Input: part model. Units: mm. Frame: model coordinates. Face numbers are marked on the shaded views. A direction names the side the tool comes from. Give positions to 0.01 mm unless a question says otherwise; leave off trailing zeros. Loops run counter-clockwise (first coordinate to the right, second up) from the corner with the lowest first, then second, coordinate; pieces in that order, holes last. Notation, with made-up numbers: (4.5, -14.5) - (24.5, -14.5) arc R9 ccw to (24.5, 0.5) - close; hole circle Ø5 at (30, 81). An arc over 180 degrees is marked (long way). Answer as a JSON object with one key per item and string values. Group by question number.
(1) Section query A-A (z = -522.75). Return loops of the section in (x, y), plus the area to 3 significant figures.
(2) Access query for the marked faces 4 and 5. Directions: +Z, -Z, +X, -X, +Y, -Y. A direction counts if a zero-diameter tool reaches every point of the face in a straight line with its end or side. Return the directions, or none.
(3) Pin query (flat end, axial travel): P1, Ø1.5, axis at y = 596, z = -512.5, coming from the +X side; P2, Ø4.5, axis at x = -734.753, z = -516, coming from the -Y side. Return the tip coordinate at first contact, or that it passes through.
(4) Section query C-C (x = -759.5). Return loops of the section in (y, z), plus the area to 3 significant figures.
(5) Section query B-B (y = 595). Return loops of the section in (x, z), plus the area to 3 significant figures.
(6) Mould query, pull axis X, two halves, no side actions, for the marked faces 1, 2 and 3. Classes: +X half, -X half, draft (parallel to the pull), parting line (faces both ways), or undercut.
(7) Section query D-D (z = -516). Return loops of the section in (x, y).
(8) Material intervals for L1, parallel to X at y = 594.95, z = -521.75; L2, parallel to X at y = 596.7, z = -516; L3, parallel to X at y = 595.7, z = -517.5, sorted ascending.
```python
from build123d import *

# Parameters (mm, degrees)
BOX001_W        = 40
BOX001_H        = 4
BOX001_DEPTH    = 25
SKETCH002_R     = 2.5781
POCKET002_DEPTH = 4.001
FILLET_R        = 10


with BuildPart() as part:
    # Box001 → Box001 (new body)
    with BuildSketch(Plane(origin=(-768, 594, -530), x_dir=(1, 0, 0), z_dir=(0, 0, 1))):
        with Locations((20, 2)):
            Rectangle(BOX001_W, BOX001_H)
    extrude(amount=BOX001_DEPTH)

    # Sketch002 → Pocket002 (cut, through all)
    with BuildSketch(Plane(origin=(-768, 598, -530), x_dir=(-1, 0, 0), z_dir=(0, 1, 0))):
        with Locations((-33.247, 14)):
            Circle(SKETCH002_R)
        with Locations((-8.5, 14)):
            Circle(SKETCH002_R)
        with BuildLine():
            ThreePointArc((-13.7, 12), (-20.85, 19.15), (-28, 12))
            Line((-28, 12), (-28, 0))
            Line((-28, 0), (-13.7, 0))
            Line((-13.7, 12), (-13.7, 0))
        make_face()
    extrude(amount=-POCKET002_DEPTH, mode=Mode.SUBTRACT)

    # Fillet
    fillet_edges = [part.edges().sort_by_distance(p)[0] for p in [
        (-728, 596, -505),
    ]]
    fillet(fillet_edges, radius=FILLET_R)


solid = part.part
```
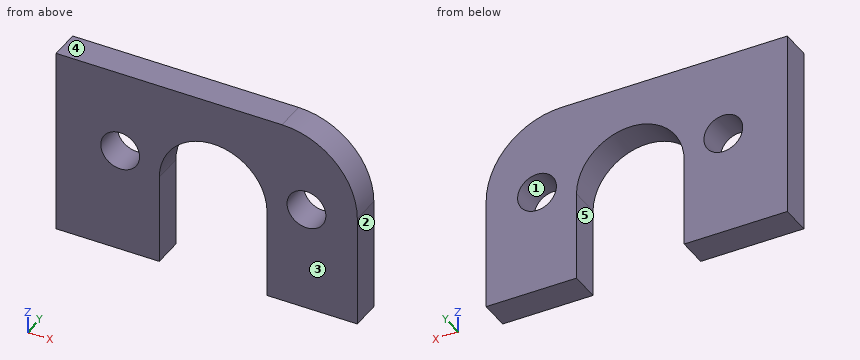
Recorded:
{
 "1": {"outline": "(-768, 594) - (-754.3, 594) - (-754.3, 598) - (-768, 598) - close; (-740, 594) - (-728, 594) - (-728, 598) - (-740, 598) - close", "area": "103 mm^2"},
 "2": {"face 4": "+Z, +X, -X, +Y, -Y", "face 5": "-Z, +Y, -Y"},
 "3": {"P1": "stops at x = -728.15", "P2": "passes through"},
 "4": {"outline": "(594, -530) - (598, -530) - (598, -518.58) - (594, -518.58) - close; (594, -513.42) - (598, -513.42) - (598, -505) - (594, -505) - close", "area": "79.4 mm^2"},
 "5": {"outline": "(-768, -530) - (-754.3, -530) - (-754.3, -518) arc R7.15 cw to (-740, -518) - (-740, -530) - (-728, -530) - (-728, -515) arc R10 ccw to (-738, -505) - (-768, -505) - close; hole circle Ø5.16 at (-759.5, -516); hole circle Ø5.16 at (-734.75, -516)", "area": "685 mm^2"},
 "6": {"face 1": "undercut", "face 2": "+X half", "face 3": "draft"},
 "7": {"outline": "(-768, 594) - (-762.08, 594) - (-762.08, 598) - (-768, 598) - close; (-756.92, 594) - (-754.01, 594) - (-754.01, 598) - (-756.92, 598) - close; (-740.29, 594) - (-737.33, 594) - (-737.33, 598) - (-740.29, 598) - close; (-732.17, 594) - (-728, 594) - (-728, 598) - (-732.17, 598) - close"},
 "8": {"L1": "x = -768 to -754.3, -740 to -728", "L2": "x = -768 to -762.08, -756.92 to -754.01, -740.29 to -737.33, -732.17 to -728", "L3": "x = -768 to -761.6, -757.4 to -754.28, -740.02 to -736.85, -732.66 to -728"}
}
